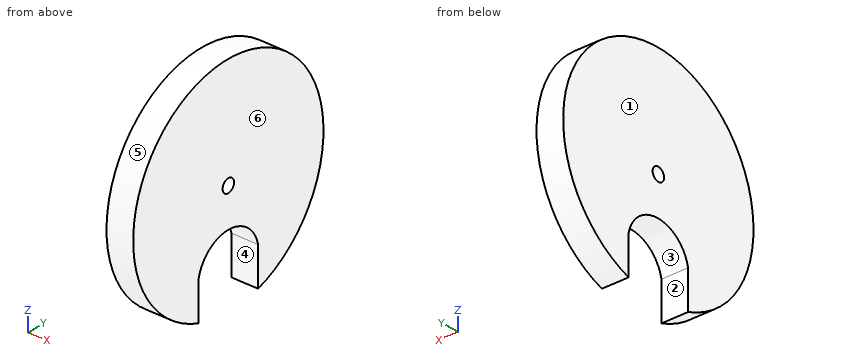
from build123d import *

# Parameters (mm, degrees)
SKETCH_R  = 3
PAD_DEPTH = 12


with BuildPart() as part:
    # Sketch → Pad (new body)
    with BuildSketch(Plane.YZ):
        with BuildLine():
            ThreePointArc((15.646539, -47.488797), (0, 50), (-15.646539, -47.488797))
            Line((-15.646539, -30.053604), (-15.646539, -47.488797))
            ThreePointArc((15.646539, -30.053604), (0, -17.398124), (-15.646539, -30.053604))
            Line((15.646539, -47.488797), (15.646539, -30.053604))
        make_face()
        Circle(SKETCH_R, mode=Mode.SUBTRACT)
    extrude(amount=PAD_DEPTH)


solid = part.part
Source: CAD feature listing. Evaluate the final solid. Frame: model axes, mm. Face numbers are marked on the shaded views. A direction names the side the tool comes from. Coordinates: 2 decimals unless noted, no trailing zeros. Loops run counter-clockwise (first coordinate to the right, second up) from the corner with the lowest first, then second, coordinate; pieces in that order, holes last. Notation, with made-up numbers: (6.5, -15) -> (43.5, -15) arc R13 ccw to (43.5, -1) -> close; hole circle Ø4 at (-35, 36.5). An arc over 180 degrees is marked (long way). Answer in a Markdown table with one row per item. Add a question column.
Q1. Section B-B on y = 0. Return the cut outline in (x, z).
Q2. Pull-direction query (Y, two-part tool) for the marked faces 3, 4, 5 and 6; classes: pulls with the +Y half, pulls with the -Y half, needs draft (parallel to the pull), parting line crosses it, or undercut.
Q3. Section C-C on x = 10. Return the cut outline in (y, z), and give its area (3 significant figures).
Q4. Section D-D on y = -18. Return the cut outline in (x, z), and give its area (3 significant figures).
Q5. Section A-A on z = 0. Return the cut outline in (x, y).
Q6. Contact query for flat-ended pins moving along their axis: pin 1 Ø6 at (x, z) = (10.5, -30) entering from +Y; pin 2 Ø6 at (x, z) = (3.5, -41.5) entering from +Y; pin 3 Ø1 at (x, z) = (5.5, 13) entering from +Y; pin 4 Ø9.5 at (y, z) = (0, 0) entering from +X. Output: stop coordinate, or through.
Q7. Ray query, line 1 along Z through (x, y) = (7.75, 0); line 2 along Y through (x, z) = (5.5, -35.5); line 3 along Y through (x, z) = (10.5, -38). Return the intervals inside material, ascending.
Q8. Reachability of the marked faces 1 and 2 from +Z, -Z, +X, -X, +Y, -Y: full face, straight path, thin tool, end or side. Return the list, or none.
Computed values:
| question | item | result |
|---|---|---|
| 1 | outline | (0, -17.4) -> (12, -17.4) -> (12, -3) -> (0, -3) -> close; (0, 3) -> (12, 3) -> (12, 50) -> (0, 50) -> close |
| 2 | face 3 | undercut |
| 2 | face 4 | undercut |
| 2 | face 5 | parting line crosses it |
| 2 | face 6 | needs draft |
| 3 | outline | (-15.65, -47.49) -> (-15.65, -30.05) arc R16 cw to (15.65, -30.05) -> (15.65, -47.49) arc R50 ccw (long way) to start; hole circle Ø6 at (0, 0) |
| 3 | area | 6,930 mm^2 |
| 4 | outline | (0, -46.65) -> (12, -46.65) -> (12, 46.65) -> (0, 46.65) -> close |
| 4 | area | 1,120 mm^2 |
| 5 | outline | (0, -50) -> (12, -50) -> (12, -3) -> (0, -3) -> close; (0, 3) -> (12, 3) -> (12, 50) -> (0, 50) -> close |
| 6 | pin 1 | stops at y = 42.08 |
| 6 | pin 2 | stops at y = 31.9 |
| 6 | pin 3 | stops at y = 48.41 |
| 6 | pin 4 | stops at x = 12 |
| 7 | line 1 | z = -17.4 to -3, 3 to 50 |
| 7 | line 2 | y = -35.21 to -15.65, 15.65 to 35.21 |
| 7 | line 3 | y = -32.5 to -15.65, 15.65 to 32.5 |
| 8 | face 1 | +Z, -Z, -X, +Y, -Y |
| 8 | face 2 | -Z, +X, -X |
